```python
from build123d import *

# Parameters (mm, degrees)
F0_R     = 1.7
F1_DEPTH = 3
F0_R_2   = 4.7
F0_R_3   = 2.7
F2_DEPTH = 6
F3_DEPTH = 2
F4_SIZE  = 2.99999
F5_START = 2
F5_DEPTH = 0.3


# Not quite as in the source:
# - a fillet or chamfer is up to 0.001 mm smaller than in the source, because OpenCascade refuses the exact size


with BuildPart() as f1:
    # F0 (on Top) → F1 (new body)
    with BuildSketch(Plane.XY):
        Polygon((12.5, 19), (-12.5, 19), (-60, 19), (-60, 7.5), (-12.5, 7.5), (12.5, 7.5), (60, 7.5), (60, 19), align=None)
        with Locations((0, 14)):
            Circle(F0_R, mode=Mode.SUBTRACT)
    extrude(amount=F1_DEPTH)



with BuildPart() as f1b:
    # F0 (on Top) → F1, piece 2 (new body)
    with BuildSketch(Plane.XY):
        Polygon((-12.5, -7.5), (-60, -7.5), (-60, -19), (-8.9196664095, -19), (8.9196664095, -19), (16.0803335905, -19), (60, -19), (60, -7.5), (12.5, -7.5), align=None)
        with Locations((0, -14)):
            Circle(F0_R, mode=Mode.SUBTRACT)
    extrude(amount=F1_DEPTH)


with BuildPart() as f1_1:
    add(f1.part)

    add(f1b.part)  # F2 merges F1b
    # F0 (on Top) → F2 (join)
    with BuildSketch(Plane.XY):
        Polygon((-12.5, 7.5), (-60, 7.5), (-60, -7.5), (-12.5, -7.5), (12.5, -7.5), (60, -7.5), (60, 7.5), (12.5, 7.5), align=None)
        with Locations((-50, 0)):
            Circle(F0_R_2, mode=Mode.SUBTRACT)
        with Locations((50, 0)):
            Circle(F0_R_2, mode=Mode.SUBTRACT)
        with Locations((-50, 0)):
            Circle(F0_R_2)
        with Locations((-50, 0)):
            Circle(F0_R_3, mode=Mode.SUBTRACT)
        with Locations((50, 0)):
            Circle(F0_R_2)
        with Locations((50, 0)):
            Circle(F0_R_3, mode=Mode.SUBTRACT)
    extrude(amount=F2_DEPTH)

    # F0 (on Top) → F3 (cut)
    with BuildSketch(Plane.XY):
        with Locations((-50, 0)):
            Circle(F0_R_2)
        with Locations((-50, 0)):
            Circle(F0_R_3, mode=Mode.SUBTRACT)
        with Locations((50, 0)):
            Circle(F0_R_2)
        with Locations((50, 0)):
            Circle(F0_R_3, mode=Mode.SUBTRACT)
    extrude(amount=F3_DEPTH, mode=Mode.SUBTRACT)

    # F4 (size 3 in the source; OpenCascade refuses exactly that, so slightly less here)
    f4_edges = [f1_1.edges().sort_by_distance(p)[0] for p in [
        (0, 7.5, 3),
        (0, -7.5, 3),
        (-60, -19, 1.5),
        (-60, 19, 1.5),
        (60, -19, 1.5),
        (60, 19, 1.5),
    ]]
    chamfer(f4_edges, length=F4_SIZE)

    # F0 (on Top) → F5 (join)
    with BuildSketch(Plane.XY.offset(F5_START)):
        with Locations((-50, 0)):
            Circle(F0_R_3)
        with Locations((50, 0)):
            Circle(F0_R_3)
    extrude(amount=F5_DEPTH)


solid = f1_1.part
```
Could you check a few things on this model? Use its own coordinates, in mm. A direction names the side the tool comes from. Round coordinates to 2 decimals unless told otherwise and drop trailing zeros. Loops run counter-clockwise (first coordinate to the right, second up) from the corner with the lowest first, then second, coordinate; pieces in that order, holes last.
Q1. Please list where these lines run through material, in increasing order: L1, parallel to Y at x = 0, z = 0.8; L2, parallel to Y at x = -50, z = 0.95; L3, parallel to X at y = 3, z = 0.3.
Q2. On a 3-axis mill with a long thin cutter (end or side, diameter ignored), from which of +Z, -Z, +X, -X, +Y, -Y can I reach the whole of each face in a straight line? I mean faces 1 (the flat face through (-1, -16, 3)), 2 (the flat face through (50, 0, 2)), 3 (the flat face through (50, 0, 2.3)). Say none if no direction works.
Q3. I want a section at C-C (y = 14). Write out the boundary of the cut face in (x, z), and give its area (3 significant figures).
Q4. For P1, Ø2.5, axis at x = -49.5, y = 0.5, coming from the +Z side; P2, Ø7, axis at x = 24.5, y = 13.5, coming from the +Z side; P3, Ø5.5, axis at x = 50, y = 0, coming from the -Z side, each with a flat end and sliding along its axis, tell me the tip position at first contact or that it passes through.
Q5. I want a section at A-A (x = 0). Give the number of separate pieces and of enclosed holes in the cut face, and give its area (3 significant figures).
Q6. Thinking about a two-plate mould opening in Y: for faces 4 (the cylindrical face through (-54.695, 0.207, 0.986)), 5 (the flat face through (59, 17, 1)), 6 (the cylindrical face through (45.305, 0.207, 0.986)), 7 (the flat face through (0.8, -9, 4.5)), which applies, pulls with the +Y half, pulls with the -Y half, needs draft (parallel to the pull), parting line crosses it, or undercut?
Q7. I want a section at B-B (z = 0.9). Write out the boundary of the cut face in (x, y).
Answer below:
1. L1: y = -19 to -15.7, -12.3 to 12.3, 15.7 to 19
1. L2: y = -19 to -4.7, 4.7 to 19
1. L3: x = -60 to -53.62, -46.38 to 46.38, 53.62 to 60
2. face 1: +Z, +X, -X, -Y
2. face 2: -Z
2. face 3: +Z
3. outline: (-60, 0) - (-1.7, 0) - (-1.7, 3) - (-60, 3) - close; (1.7, 0) - (60, 0) - (60, 3) - (1.7, 3) - close
3. area: 350 mm2
4. P1: stops at z = 2.3
4. P2: stops at z = 3.5
4. P3: stops at z = 2
5. separate pieces: 3
5. enclosed holes: 0
5. area: 148 mm2
6. face 4: undercut
6. face 5: pulls with the +Y half
6. face 6: undercut
6. face 7: pulls with the -Y half
7. outline: (-60, -16) - (-57, -19) - (57, -19) - (60, -16) - (60, 16) - (57, 19) - (-57, 19) - (-60, 16) - close; hole circle Ø9.4 at (-50, 0); hole circle Ø3.4 at (0, -14); hole circle Ø3.4 at (0, 14); hole circle Ø9.4 at (50, 0)
